from build123d import *

# Parameters (mm, degrees)
SKETCH_1_W              = 80
SKETCH_1_H              = 34
EXTRUDE_1_DEPTH         = 3
SKETCH_2_W              = 70
SKETCH_2_H              = 23
CUT_EXTRUDE_2_DEPTH     = 3
CHAMFER_1_SIZE          = 0.5
SKETCH_7_W              = 25
SKETCH_7_H              = 3
CUT_EXTRUDE_6_DEPTH     = 3
FILLET_2_R              = 2
CHAMFER_2_SIZE          = 11
CHAMFER_2_SIZE2         = 6.350852961
CHAMFER_3_SIZE          = 11
CHAMFER_3_SIZE2         = 6.350852961
FILLET_3_R              = 2
HOLE_WIZARD_2_5_2_5_1_D = 2.5


with BuildPart() as part:
    # 草图1 → Extrude 1 (new body)
    with BuildSketch(Plane.XY):
        Rectangle(SKETCH_1_W, SKETCH_1_H)
    extrude(amount=EXTRUDE_1_DEPTH)

    # 草图2 → 拉伸2 (cut)
    with BuildSketch(Plane.XY.offset(3)):
        Rectangle(SKETCH_2_W, SKETCH_2_H)
    extrude(amount=-CUT_EXTRUDE_2_DEPTH, mode=Mode.SUBTRACT)

    # 倒角1
    chamfer_1_edges = [part.edges().sort_by_distance(p)[0] for p in [
        (-40, 17, 1.5),
        (40, 17, 1.5),
    ]]
    chamfer(chamfer_1_edges, length=CHAMFER_1_SIZE)

    # 草图7 → 拉伸6 (cut)
    with BuildSketch(Plane.XY.offset(3)):
        with Locations((0, -15.5)):
            Rectangle(SKETCH_7_W, SKETCH_7_H)
    extrude(amount=-CUT_EXTRUDE_6_DEPTH, mode=Mode.SUBTRACT)

    # 圆角2
    fillet_2_edges = [part.edges().sort_by_distance(p)[0] for p in [
        (-12.5, -14, 1.5),
        (12.5, -14, 1.5),
    ]]
    fillet(fillet_2_edges, radius=FILLET_2_R)

    # 倒角2
    chamfer_2_edges = [part.edges().sort_by_distance(p)[0] for p in [
        (40, -17, 1.5),
    ]]
    chamfer_2_side = [part.faces().sort_by_distance(p)[0] for p in [
        (26.25, -17, 1.5),
    ]]
    chamfer(chamfer_2_edges, length=CHAMFER_2_SIZE, length2=CHAMFER_2_SIZE2, reference=chamfer_2_side[0])

    # 倒角3
    chamfer_3_edges = [part.edges().sort_by_distance(p)[0] for p in [
        (-40, -17, 1.5),
    ]]
    chamfer_3_side = [part.faces().sort_by_distance(p)[0] for p in [
        (-26.25, -17, 1.5),
    ]]
    chamfer(chamfer_3_edges, length=CHAMFER_3_SIZE, length2=CHAMFER_3_SIZE2, reference=chamfer_3_side[0])

    # 圆角3
    fillet_3_edges = [part.edges().sort_by_distance(p)[0] for p in [
        (12.5, -17, 1.5),
        (-12.5, -17, 1.5),
    ]]
    fillet(fillet_3_edges, radius=FILLET_3_R)

    # Ø2.5 (2.5) 直径孔1 (through all)
    with Locations(Plane(origin=(-37.5, -7, 0), x_dir=(-1, 0, 0), z_dir=(0, 0, -1))):
        with Locations((0, 0), (0, 21), (-75, 21), (-75, 0)):
            Hole(HOLE_WIZARD_2_5_2_5_1_D / 2)


solid = part.part
Model file for the job. Use its own axes, mm. A direction names the side the tool comes from. Round coordinates to 2 decimals unless told otherwise and drop trailing zeros. Order: outer loops, then holes, each group sorted by start corner. A loop starts at its lowest first (then second) coordinate and runs counter-clockwise, first axis right, second up.
(1) 3-axis set-ups, long thin cutter, end or side, ignore diameter. For faces 1 (the face through (35, 0, 2)), 2 (the face through (0, -14, 2)), 3 (the face through (0, 14, 0)): which of +Z, -Z, +X, -X, +Y, -Y reach the whole face in a straight line?
(2) Band-saw the part on B-B (y = 14). List the corners of the cut face in (x, z).
(3) Band-saw the part on A-A (x = 17.5). List the corners of the cut face in (y, z).
(4) Band-saw the part on D-D (y = 4.5). List the corners of the cut face in (x, z), then the cut area to 3 significant figures.
(5) Pin check, flat tips, straight feed: pin 1 (3 mm diameter, centred on x = 37.5, y = 14, fed in from +Z); pin 2 (0.9 mm diameter, centred on x = -4.5, z = 2, fed in from -Y). Stop position of each tip, or through.
(6) Drill centre lines: line 1 (X direction, y = -5, z = 1); line 2 (X direction, y = -8, z = 0.1); line 3 (X direction, y = 13, z = 1). Where is each one in solid material? Low to high.
(7) Band-saw the part on C-C (y = -7). List the corners of the cut face in (x, z), then the cut area to 3 significant figures.
(8) Pull direction Y, two halves, no side cores. Call faces 4 (the face through (0, 14, 3)), 5 (the face through (-34.58, -13.78, 1.48)), 6 (the face through (0, 11.5, 2)): released by +Y, released by -Y, zero draft, split by the parting line, or undercut.
Verdict:
1. face 1: +Z, -Z
1. face 2: +Z, -Z, -Y
1. face 3: -Z, +X, -X, +Y, -Y
2. outline: (-40, 0) - (-38.75, 0) - (-38.75, 3) - (-40, 3) - close; (-36.25, 0) - (36.25, 0) - (36.25, 3) - (-36.25, 3) - close; (38.75, 0) - (40, 0) - (40, 3) - (38.75, 3) - close
3. outline: (-17, 0) - (-11.5, 0) - (-11.5, 3) - (-17, 3) - close; (11.5, 0) - (17, 0) - (17, 3) - (11.5, 3) - close
4. outline: (-40, 0) - (-35, 0) - (-35, 3) - (-40, 3) - close; (35, 0) - (40, 0) - (40, 3) - (35, 3) - close
4. area: 30.0 mm2
5. pin 1: stops at z = 3
5. pin 2: stops at y = -14
6. line 1: x = -40 to -35, 35 to 40
6. line 2: x = -40 to -38.25, -36.75 to -35, 35 to 36.75, 38.25 to 40
6. line 3: x = -40 to -38.25, -36.75 to 36.75, 38.25 to 40
7. outline: (-40, 0) - (-38.75, 0) - (-38.75, 3) - (-40, 3) - close; (-36.25, 0) - (-35, 0) - (-35, 3) - (-36.25, 3) - close; (35, 0) - (36.25, 0) - (36.25, 3) - (35, 3) - close; (38.75, 0) - (40, 0) - (40, 3) - (38.75, 3) - close
7. area: 15.0 mm2
8. face 4: zero draft
8. face 5: released by -Y
8. face 6: undercut
